from build123d import *

# Parameters (mm, degrees)
F0_W     = 54
F0_H     = 54
F1_DEPTH = 120
F2_W     = 60
F2_H     = 60
F2_R     = 6
F3_DEPTH = 6
F4_W     = 20
F4_H     = 120
F5_DEPTH = 6


with BuildPart() as f1:
    # F0 (on Front) → F1 (new body)
    with BuildSketch(Plane.XZ):
        with BuildLine():
            ThreePointArc((30, 25), (28.5355339059, 28.5355339059), (25, 30))
            Line((25, 30), (-25, 30))
            ThreePointArc((-25, 30), (-28.5355339059, 28.5355339059), (-30, 25))
            Line((-30, 25), (-30, -25))
            ThreePointArc((-30, -25), (-28.5355339059, -28.5355339059), (-25, -30))
            Line((-25, -30), (25, -30))
            ThreePointArc((25, -30), (28.5355339059, -28.5355339059), (30, -25))
            Line((30, -25), (30, 25))
        make_face()
        Rectangle(F0_W, F0_H, mode=Mode.SUBTRACT)
    extrude(amount=F1_DEPTH)

    # F2 (on face) → F3 (join)
    with BuildSketch(Plane.XZ.offset(120)):
        Rectangle(F2_W, F2_H)
        Circle(F2_R, mode=Mode.SUBTRACT)
    extrude(amount=-F3_DEPTH)

    # F4 (on face) → F5 (join)
    with BuildSketch(Plane(origin=(0, 0, -30), x_dir=(1, 0, 0), z_dir=(0, 0, -1))):
        with Locations((40, 60)):
            Rectangle(F4_W, F4_H)
        with Locations((-40, 60)):
            Rectangle(F4_W, F4_H)
    extrude(amount=-F5_DEPTH)


solid = f1.part
Model file for the job. Use its own axes, mm. A direction names the side the tool comes from. Give positions to 0.01 mm unless a question says otherwise; leave off trailing zeros. Loops run counter-clockwise (first coordinate to the right, second up) from the corner with the lowest first, then second, coordinate; pieces in that order, holes last.
1) Pull direction Z, two halves, no side cores. Call faces 1 (the flat face through (27, -56, 0)), 2 (the cylindrical face through (-28, -56, 29)), 3 (the flat face through (3, 0, -29)): +Z half, -Z half, draft (parallel to the pull), parting line (faces both ways), or undercut.
2) Tool access for faces 4 (the flat face through (-29, -114, -29)), 5 (the flat face through (-40, -61, -24)), 6 (the flat face through (-6.4, -114, 0.4)): list every direction of +Z, -Z, +X, -X, +Y, -Y with a clear straight run to the whole face (end or side of a thin tool).
3) Flat gauge pins, fed straight in: pin 1 Ø4 at (y, z) = (-31, 4.5) entering from -X; pin 2 Ø16 at (y, z) = (-85.5, 4.5) entering from +X; pin 3 Ø10 at (x, y) = (-36.5, -77.5) entering from +Z. Where does each tip first touch, or does it go through?
4) Saw through at C-C (y = -22.5). Write the cut outline in (x, z), plus the area to 3 significant figures.
5) Saw through at D-D (x = 18). Write the cut outline in (y, z).
6) Saw through at A-A (z = 0). Write the cut outline in (x, y).
7) Saw through at B-B (x = 0). Write the cut outline in (y, z).
8) Wall check: line 1 (X direction, y = -86, z = 1); line 2 (Z direction, x = 0, y = -117.6). Give the ranges that are in metal, low to high.
Answer block:
1. face 1: undercut
1. face 2: +Z half
1. face 3: draft
2. face 4: -Z, +Y
2. face 5: +Z, -X, +Y, -Y
2. face 6: +Y
3. pin 1: stops at x = -30
3. pin 2: stops at x = 30
3. pin 3: stops at z = -24
4. outline: (-50, -30) - (-30, -30) - (-30, -25) arc R5 ccw to (-25, -30) - (25, -30) arc R5 ccw to (30, -25) - (30, -30) - (50, -30) - (50, -24) - (30, -24) - (30, 25) arc R5 ccw to (25, 30) - (-25, 30) arc R5 ccw to (-30, 25) - (-30, -24) - (-50, -24) - close; hole (-27, -27) - (27, -27) - (27, 27) - (-27, 27) - close
4. area: 903 mm2
5. outline: (-120, -30) - (0, -30) - (0, -27) - (-114, -27) - (-114, 27) - (0, 27) - (0, 30) - (-120, 30) - close
6. outline: (-30, -120) - (-6, -120) - (-6, -114) - (-27, -114) - (-27, 0) - (-30, 0) - close; (6, -120) - (30, -120) - (30, 0) - (27, 0) - (27, -114) - (6, -114) - close
7. outline: (-120, -30) - (0, -30) - (0, -27) - (-114, -27) - (-114, -6) - (-120, -6) - close; (-120, 6) - (-114, 6) - (-114, 27) - (0, 27) - (0, 30) - (-120, 30) - close
8. line 1: x = -30 to -27, 27 to 30
8. line 2: z = -30 to -6, 6 to 30
